CAD build for the part. Positions are in the model's coordinates, mm. Round coordinates to 2 decimals unless told otherwise and drop trailing zeros. Order: outer loops, then holes, each group sorted by start corner. A loop starts at its lowest first (then second) coordinate and runs counter-clockwise, first axis right, second up. Notation, with made-up numbers: M 37.5,-20 L 51.5,-20 A20 cw 51.5,-12 Z; hole C 26,87.5 d11. An arc over 180 degrees is marked long. Answer as a JSON object with one key per item and string values.
```python
from build123d import *

# Parameters (mm, degrees)
SKETCH1_W           = 17.5
SKETCH1_H           = 25
SKETCH1_W_2         = 50
BOSS_EXTRUDE1_DEPTH = 5
SKETCH2_R           = 11.25
CUT_EXTRUDE1_DEPTH  = 2.5
SKETCH3_R           = 1
SKETCH3_R_2         = 3.5
CUT_EXTRUDE2_DEPTH  = 5
SKETCH4_R           = 5
CUT_EXTRUDE3_DEPTH  = 5
CUT_EXTRUDE4_DEPTH  = 5
CHAMFER3_SIZE       = 1.5
BOSS_EXTRUDE2_DEPTH = 5
CHAMFER4_SIZE       = 2.5
CUT_EXTRUDE11_DEPTH = 5
SKETCH10_R          = 2.5
CUT_EXTRUDE13_DEPTH = 5
CHAMFER5_SIZE       = 5
CHAMFER5_SIZE_2     = 7.280109889
CHAMFER5_SIZE_3     = 5.321683239
FILLET1_R           = 5
SKETCH12_R          = 7.5
CUT_EXTRUDE14_DEPTH = 2.5


# Some blends are built 0.0001 mm under size
with BuildPart() as part:
    # Sketch1 → Boss-Extrude1 (new body)
    with BuildSketch(Plane.XY):
        with Locations((-33.75, 0)):
            Rectangle(SKETCH1_W, SKETCH1_H)
        Polygon((-25, -12.5), (-42.5, -12.5), (-42.5, 12.5), (-25, 12.5), (-25, 17.5), (-60, 17.5), (-60, -17.5), (-25, -17.5), align=None)
        Rectangle(SKETCH1_W_2, SKETCH1_H)
        with Locations((33.75, 0)):
            Rectangle(SKETCH1_W, SKETCH1_H)
        Polygon((42.5, -12.5), (25, -12.5), (25, -17.5), (60, -17.5), (60, 17.5), (25, 17.5), (25, 12.5), (42.5, 12.5), align=None)
    extrude(amount=BOSS_EXTRUDE1_DEPTH)

    # Sketch2 → Cut-Extrude1 (cut)
    with BuildSketch(Plane.XY.offset(5)):
        with Locations((-42.5, 0)):
            Circle(SKETCH2_R)
        with Locations((42.5, 0)):
            Circle(SKETCH2_R)
    extrude(amount=-CUT_EXTRUDE1_DEPTH, mode=Mode.SUBTRACT)

    # Sketch3 → Cut-Extrude2 (cut)
    with BuildSketch(Plane.XY.offset(2.5)):
        with Locations((42.5, 7)):
            Circle(SKETCH3_R)
        with Locations((46, 7)):
            Circle(SKETCH3_R)
        with Locations((39, 7)):
            Circle(SKETCH3_R)
        with Locations((42.5, 0)):
            Circle(SKETCH3_R_2)
        with Locations((-42.5, 0)):
            Circle(SKETCH3_R_2)
        with Locations((-39, 7)):
            Circle(SKETCH3_R)
        with Locations((-46, 7)):
            Circle(SKETCH3_R)
        with Locations((-42.5, 7)):
            Circle(SKETCH3_R)
        with Locations((49.5, 0)):
            Circle(SKETCH3_R)
        with Locations((49.5, -3.5)):
            Circle(SKETCH3_R)
        with Locations((49.5, 3.5)):
            Circle(SKETCH3_R)
        with Locations((42.5, -7)):
            Circle(SKETCH3_R)
        with Locations((39, -7)):
            Circle(SKETCH3_R)
        with Locations((46, -7)):
            Circle(SKETCH3_R)
        with Locations((35.5, 0)):
            Circle(SKETCH3_R)
        with Locations((35.5, 3.5)):
            Circle(SKETCH3_R)
        with Locations((35.5, -3.5)):
            Circle(SKETCH3_R)
        with Locations((-35.5, 3.5)):
            Circle(SKETCH3_R)
        with Locations((-35.5, 0)):
            Circle(SKETCH3_R)
        with Locations((-35.5, -3.5)):
            Circle(SKETCH3_R)
        with Locations((-39, -7)):
            Circle(SKETCH3_R)
        with Locations((-42.5, -7)):
            Circle(SKETCH3_R)
        with Locations((-46, -7)):
            Circle(SKETCH3_R)
        with Locations((-49.5, -3.5)):
            Circle(SKETCH3_R)
        with Locations((-49.5, 0)):
            Circle(SKETCH3_R)
        with Locations((-49.5, 3.5)):
            Circle(SKETCH3_R)
    extrude(amount=-CUT_EXTRUDE2_DEPTH, mode=Mode.SUBTRACT)

    # Sketch4 → Cut-Extrude3 (cut)
    with BuildSketch(Plane.XY.offset(5)):
        Circle(SKETCH4_R)
    extrude(amount=-CUT_EXTRUDE3_DEPTH, mode=Mode.SUBTRACT)

    # Sketch5 → Cut-Extrude4 (cut)
    with BuildSketch(Plane.XY.offset(5)):
        Polygon((20.600480947, -6.120190528), (21.899519053, -6.870190528), (29.399519053, 6.120190528), (28.100480947, 6.870190528), align=None)
        Polygon((15.600480947, -6.120190528), (23.100480947, 6.870190528), (24.399519053, 6.120190528), (16.899519053, -6.870190528), align=None)
        Polygon((10.600480947, -6.120190528), (18.100480947, 6.870190528), (19.399519053, 6.120190528), (11.899519053, -6.870190528), align=None)
        Polygon((-19.399519053, -6.120190528), (-11.899519053, 6.870190528), (-10.600480947, 6.120190528), (-18.100480947, -6.870190528), align=None)
        Polygon((-24.399519053, -6.120190528), (-16.899519053, 6.870190528), (-15.600480947, 6.120190528), (-23.100480947, -6.870190528), align=None)
        Polygon((-29.399519053, -6.120190528), (-21.899519053, 6.870190528), (-20.600480947, 6.120190528), (-28.100480947, -6.870190528), align=None)
    extrude(amount=-CUT_EXTRUDE4_DEPTH, mode=Mode.SUBTRACT)

    # Chamfer3
    chamfer3_edges = [part.edges().sort_by_distance(p)[0] for p in [
        (39, 0, 0),
        (-46, 0, 0),
    ]]
    chamfer(chamfer3_edges, length=CHAMFER3_SIZE)

    # Sketch7 → Boss-Extrude2 (add)
    with BuildSketch(Plane(origin=(0, 0, 0), x_dir=(-1, 0, 0), z_dir=(0, 0, -1))):
        Polygon((-25, 27.5), (-60, 17.5), (-25, 17.5), (-25, 12.5), (25, 12.5), (25, 17.5), (60, 17.5), (60, 22.5), align=None)
    extrude(amount=-BOSS_EXTRUDE2_DEPTH)

    # Chamfer4
    chamfer4_edges = [part.edges().sort_by_distance(p)[0] for p in [
        (-42.5, -17.5, 0),
        (-60, 2.5, 0),
        (60, 0, 0),
        (42.5, -17.5, 0),
        (25, -15, 0),
        (0, -12.5, 0),
        (-25, -15, 0),
        (-25, -17.5, 2.5),
        (25, -17.5, 2.5),
        (25, -12.5, 2.5),
        (-25, -12.5, 2.5),
        (42.5, 22.5, 0),
        (-17.5, 25, 0),
    ]]
    chamfer(chamfer4_edges, length=CHAMFER4_SIZE - 0.0001)  # a hair under: the kernel refuses the full size

    # Sketch8 → Cut-Extrude11 (cut)
    with BuildSketch(Plane.XY.offset(5)):
        with BuildLine():
            Line((-22.5, 17.5), (22.5, 17.5))
            ThreePointArc((22.5, 17.5), (25, 15), (22.5, 12.5))
            Line((22.5, 12.5), (-22.5, 12.5))
            ThreePointArc((-22.5, 12.5), (-25, 15), (-22.5, 17.5))
        make_face()
    extrude(amount=-CUT_EXTRUDE11_DEPTH, mode=Mode.SUBTRACT)

    # Sketch10 → Cut-Extrude13 (cut)
    with BuildSketch(Plane.XY.offset(5)):
        with Locations((-52.5, -11)):
            Circle(SKETCH10_R)
        with Locations((53, -11.5)):
            Circle(SKETCH10_R)
        with Locations(Location((53, 11.5, 0), (0, 0, 180))):
            Circle(SKETCH10_R)
        with Locations(Location((-52.5, 16, 0), (0, 0, 180))):
            Circle(SKETCH10_R)
    extrude(amount=-CUT_EXTRUDE13_DEPTH, mode=Mode.SUBTRACT)

    # Chamfer5
    # the kernel refuses this chamfer: 7.280109889, 5.321683239, 5 mm, written as the material it takes off along each edge
    with BuildSketch(Plane(origin=(-60, -17.5, -10.35851494), x_dir=(0.9996219169112968, -0.027495876610586317, 0), z_dir=(0, 0, 1)), Plane(origin=(60, -17.5, -10.35851494), x_dir=(0.027495876610586317, 0.9996219169112968, 0), z_dir=(0, 0, 1))) as chamfer5_piece_1:
        Polygon((CHAMFER5_SIZE * 0.999621916911, CHAMFER5_SIZE * 0.0274958766106), (-CHAMFER5_SIZE * 0.0274958766106, CHAMFER5_SIZE * 0.999621916911), (0, 0), align=None)
    extrude(amount=28.21692988, mode=Mode.SUBTRACT)
    with BuildSketch(Plane(origin=(60, 17.5, -16.34008853), x_dir=(-0.9561991759280333, 0.2927168187080304, 0), z_dir=(0, 0, 1))) as chamfer5_piece_2:
        Polygon((CHAMFER5_SIZE_2 * 0.999823900998, CHAMFER5_SIZE_2 * 0.0187661149602), (-CHAMFER5_SIZE * 0.292716818708, CHAMFER5_SIZE * 0.956199175928), (0, 0), align=None)
    extrude(amount=40.18007706, mode=Mode.SUBTRACT)
    with BuildSketch(Plane(origin=(-60, 22.5, -11.206616296), x_dir=(-0.02579454785928718, -0.9996672652941752, 0), z_dir=(0, 0, 1))) as chamfer5_piece_3:
        Polygon((CHAMFER5_SIZE_3 * 0.99966726536, CHAMFER5_SIZE_3 * 0.025794547861), (-CHAMFER5_SIZE * 0.0844525191923, CHAMFER5_SIZE * 0.996427504639), (0, 0), align=None)
    extrude(amount=29.913132593, mode=Mode.SUBTRACT)

    # Fillet1
    # the kernel refuses this fillet: 5 mm, written as the material it takes off along each edge
    with BuildSketch(Plane(origin=(-64.166666667, -8.333333333, 6.666566667), x_dir=(0.40824829046408034, 0.8164965809275085, -0.4082482904640807), z_dir=(0.5773502691894717, -0.5773502691899334, -0.5773502691894724)), Plane(origin=(53.333433333, 19.166566667, -4.166666667), x_dir=(-0.4082482904639215, 0.40824829046385264, 0.8164965809277018), z_dir=(0.5773502691896591, -0.5773502691895585, 0.5773502691896599)), Plane(origin=(61.666566667, -10.833433333, -4.166666667), x_dir=(0.40824829046391753, 0.4082482904635908, 0.816496580927835), z_dir=(-0.5773502691899336, -0.5773502691894719, 0.5773502691894719))) as fillet1_piece_1:
        with BuildLine():
            CenterArc((FILLET1_R * 0.577350269189, FILLET1_R), FILLET1_R, 210, 60)
            Line((-FILLET1_R * 0.288675134595, FILLET1_R * 0.5), (0, 0))
            Line((0, 0), (FILLET1_R * 0.577350269189, 0))
        make_face()
    extrude(amount=18.763710544, mode=Mode.SUBTRACT)
    with BuildSketch(Plane(origin=(-50.833333333, -21.666666667, 6.666566667), x_dir=(0.8164965809279436, 0.4082482904636451, -0.4082482904636457), z_dir=(-0.577350269189318, 0.5773502691897797, -0.5773502691897796)), Plane(origin=(64.166666667, -8.333333333, 6.666566667), x_dir=(-0.4082482904636451, 0.8164965809279439, -0.4082482904636454), z_dir=(-0.5773502691897794, -0.5773502691893178, -0.5773502691897802)), Plane(origin=(-51.093826671, 27.197761756, 6.666566667), x_dir=(-0.38357064118824047, -0.4315169713371016, 0.8164965809276222), z_dir=(-0.5424508028963463, -0.6102571532588589, -0.5773502691897726))) as fillet1_piece_2:
        with BuildLine():
            CenterArc((FILLET1_R * 0.57735026919, -FILLET1_R), FILLET1_R, 90, 60)
            Line((-FILLET1_R * 0.288675134595, -FILLET1_R * 0.5), (0, 0))
            Line((0, 0), (FILLET1_R * 0.57735026919, 0))
        make_face()
    extrude(amount=18.763710544, mode=Mode.SUBTRACT)
    with BuildSketch(Plane(origin=(60.502410392, 11.997589608, -2.652776612), x_dir=(-0.7467824303447061, -0.364905051191258, -0.5560218568937372), z_dir=(-0.6360661543203274, 0.6360661543202165, 0.43685202833046355))) as fillet1_piece_3:
        with BuildLine():
            CenterArc((FILLET1_R * 0.485798657646, FILLET1_R), FILLET1_R, 218.179161485, 51.820838515)
            Line((-FILLET1_R * 0.300283099109, FILLET1_R * 0.381877462231), (0, 0))
            Line((0, 0), (FILLET1_R * 0.485798657646, 0))
        make_face()
    extrude(amount=17.867499102, mode=Mode.SUBTRACT)
    with BuildSketch(Plane(origin=(53, 19.5, -0.739175352), x_dir=(0.7071067811866106, -0.7071067811864844, 0), z_dir=(0, 0, 1))) as fillet1_piece_4:
        with BuildLine():
            CenterArc((FILLET1_R * 0.259126028197, -FILLET1_R), FILLET1_R, 90, 29.054604099)
            Line((-FILLET1_R * 0.226516902981, -FILLET1_R * 0.125842723878), (0, 0))
            Line((0, 0), (FILLET1_R * 0.259126028197, 0))
        make_face()
    extrude(amount=8.978250705, mode=Mode.SUBTRACT)
    with BuildSketch(Plane(origin=(60, 12.5, -2.67776953), x_dir=(-0.7071067811866102, 0.707106781186485, 0), z_dir=(0, 0, 1)), Plane(origin=(55, -17.5, -2.67776953), x_dir=(0.7071067811868306, 0.7071067811862645, 0), z_dir=(0, 0, 1)), Plane(origin=(-60, -12.5, -2.67776953), x_dir=(0.7071067811862649, -0.7071067811868301, 0), z_dir=(0, 0, 1)), Plane(origin=(-55.008628134, 22.79361011, -2.67776953), x_dir=(-0.6643638388296346, -0.7474093186839131, 0), z_dir=(0, 0, 1))) as fillet1_piece_5:
        with BuildLine():
            CenterArc((FILLET1_R * 0.414213562373, FILLET1_R), FILLET1_R, 225, 45)
            Line((-FILLET1_R * 0.292893218813, FILLET1_R * 0.292893218814), (0, 0))
            Line((0, 0), (FILLET1_R * 0.414213562373, 0))
        make_face()
    extrude(amount=12.855439059, mode=Mode.SUBTRACT)
    with BuildSketch(Plane(origin=(60, -12.5, -2.67776953), x_dir=(-0.7071067811868297, -0.7071067811862654, 0), z_dir=(0, 0, 1)), Plane(origin=(-55, -17.5, -2.67776953), x_dir=(-0.7071067811862645, 0.7071067811868306, 0), z_dir=(0, 0, 1))) as fillet1_piece_6:
        with BuildLine():
            CenterArc((FILLET1_R * 0.414213562373, -FILLET1_R), FILLET1_R, 90, 45)
            Line((-FILLET1_R * 0.292893218814, -FILLET1_R * 0.292893218814), (0, 0))
            Line((0, 0), (FILLET1_R * 0.414213562373, 0))
        make_face()
    extrude(amount=12.855439059, mode=Mode.SUBTRACT)
    with BuildSketch(Plane(origin=(-60, 17.178316761, -2.252591529), x_dir=(0.6643638388296347, 0.7474093186839131, 0), z_dir=(0, 0, 1))) as fillet1_piece_7:
        with BuildLine():
            CenterArc((FILLET1_R * 0.380199322349, -FILLET1_R), FILLET1_R, 90, 41.633539337)
            Line((-FILLET1_R * 0.284164516481, -FILLET1_R * 0.252590681316), (0, 0))
            Line((0, 0), (FILLET1_R * 0.380199322349, 0))
        make_face()
    extrude(amount=12.005083059, mode=Mode.SUBTRACT)
    with BuildSketch(Plane(origin=(-53.658288342, 24.312742376, -3.841811658), x_dir=(0.440204389240274, -0.7825855808709965, -0.44020438924027366), z_dir=(-0.5533715710926945, -0.6225430174797603, 0.5533715710926953))) as fillet1_piece_8:
        with BuildLine():
            CenterArc((FILLET1_R * 0.555404268528, FILLET1_R), FILLET1_R, 211.904040139, 58.095959861)
            Line((-FILLET1_R * 0.293530154836, FILLET1_R * 0.471501802437), (0, 0))
            Line((0, 0), (FILLET1_R * 0.555404268528, 0))
        make_face()
    extrude(amount=18.402686095, mode=Mode.SUBTRACT)

    # Sketch12 → Cut-Extrude14 (cut)
    with BuildSketch(Plane(origin=(0, 0, 0), x_dir=(-1, 0, 0), z_dir=(0, 0, -1))):
        Circle(SKETCH12_R)
    extrude(amount=-CUT_EXTRUDE14_DEPTH, mode=Mode.SUBTRACT)


solid = part.part
```
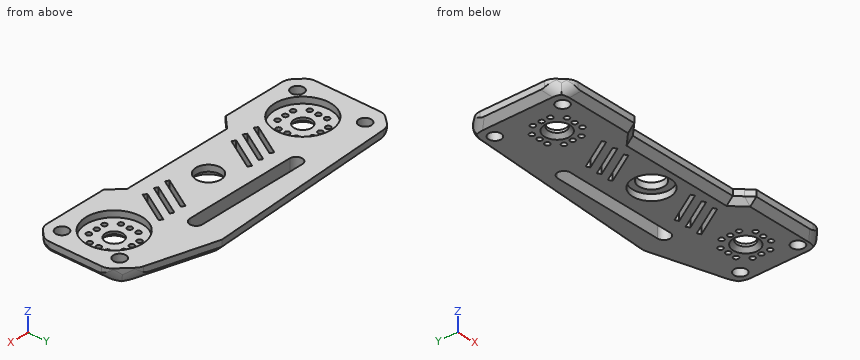
Item 1: Saw through at B-B on x = -13.5. List the corners of the cut face in (y, z).
Worked answers:
{"outline": "M -12.5,2.5 L -10,0 L 1.1,0 L 1.1,5 L -12.5,5 Z; M 4.1,0 L 12.5,0 L 12.5,5 L 4.1,5 Z; M 17.5,0 L 22.73,0 L 25.24,2.5 L 25.24,5 L 17.5,5 Z"}
Item 2: Saw through at A-A on x = 0. List the corners of the cut face in (y, z).
Worked answers:
{"outline": "M -12.5,2.5 L -10,0 L -7.5,0 L -7.5,2.5 L -5,2.5 L -5,5 L -12.5,5 Z; M 5,2.5 L 7.5,2.5 L 7.5,0 L 12.5,0 L 12.5,5 L 5,5 Z; M 17.5,0 L 23.53,0 L 26.03,2.5 L 26.03,5 L 17.5,5 Z"}
Item 3: Wall check: line 1 along Y through (x, z) = (42.5, 3); line 2 along Y through (x, z) = (-49.5, 1.35); line 3 along X through (y, z) = (16.5, 2.8). Give the ranges that are in metal, low to high. Write a range as [from, to].
Worked answers:
{"line 1": "y = [-17.5, -11.25], [11.25, 22.5]", "line 2": "y = [-16.35, -4.5], [-2.5, -1], [1, 2.5], [4.5, 21.97]", "line 3": "x = [-59.58, -54.95], [-50.05, -24.5], [24.5, 55.99]"}
Item 4: Drop flat-ended pins along their axis: pin 1 Ø2.5 at (x, y) = (-42.5, 7) entering from +Z; pin 2 Ø2 at (x, z) = (5, 4) entering from -Y; pin 3 Ø6.5 at (x, y) = (42.5, 0) entering from -Z. Give the stop position or say it passes through.
Worked answers:
{"pin 1": "stops at z = 2.5", "pin 2": "stops at y = -12.5", "pin 3": "passes through"}
